```python
from build123d import *

# Parameters (mm, degrees)
F1_DEPTH = 25.4
F2_W     = 20.0148001313
F2_H     = 42.0691836625
F3_DEPTH = 25.4


with BuildPart() as f1:
    # F0 (on Top) → F1 (new body)
    with BuildSketch(Plane.XY):
        with BuildLine():
            Line((2.726720646, 50.0040240586), (2.726720646, -58.5763193667))
            Line((2.726720646, -58.5763193667), (62.9542395473, -58.5763193667))
            Line((62.9542395473, -58.5763193667), (62.9542395473, 27.6013473304))
            ThreePointArc((62.9542395473, 27.6013473304), (47.113154916, 34.1629394274), (40.5515628191, 50.0040240586))
            Line((40.5515628191, 50.0040240586), (2.726720646, 50.0040240586))
        make_face()
        with BuildLine():
            ThreePointArc((40.5515628191, 50.0040240586), (47.113154916, 34.1629394274), (62.9542395473, 27.6013473304))
            Line((62.9542395473, 27.6013473304), (62.9542395473, 50.0040240586))
            Line((62.9542395473, 50.0040240586), (40.5515628191, 50.0040240586))
        make_face()
        with BuildLine():
            Line((62.9542395473, 50.0040240586), (62.9542395473, 27.6013473304))
            ThreePointArc((62.9542395473, 27.6013473304), (78.7953241785, 34.1629394274), (85.3569162754, 50.0040240586))
            ThreePointArc((85.3569162754, 50.0040240586), (62.9542395473, 72.4067007867), (40.5515628191, 50.0040240586))
            Line((40.5515628191, 50.0040240586), (62.9542395473, 50.0040240586))
        make_face()
    extrude(amount=F1_DEPTH)

    # F2 (on face) → F3 (join)
    with BuildSketch(Plane.XY.offset(25.4)):
        with Locations((44.1186800599, 3.4223971888)):
            Rectangle(F2_W, F2_H)
    extrude(amount=F3_DEPTH)


solid = f1.part
```
Geometry: final body of the model. Coordinates: model frame, mm. A direction names the side the tool comes from. Coordinates: 2 decimals unless noted, no trailing zeros. Order: outer loops, then holes, each group sorted by start corner. A loop starts at its lowest first (then second) coordinate and runs counter-clockwise, first axis right, second up. Notation, with made-up numbers: (-12, -27) - (44, -27) arc R26 ccw to (44, -8) - close; hole circle Ø5 at (1.5, 61.25). An arc over 180 degrees is marked (long way). Write each question's results on one line, items separated by ' | '.
1) Pin query (flat end, axial travel): pin 1 (10 mm diameter, centred on x = 72.5, z = 7, fed in from -Y); pin 2 (12 mm diameter, centred on x = 32, y = -45, fed in from +Z); pin 3 (8 mm diameter, centred on y = -23, z = 38.5, fed in from -X); pin 4 (1 mm diameter, centred on x = 71.5, z = 12, fed in from +Y). Return the tip coordinate at first contact, or that it passes through.
Results list:
pin 1: y = 28.07 | pin 2: z = 25.4 | pin 3: through | pin 4: y = 70.91
2) Set-up query: faces 1 (the flat face through (54.126, 3, 38)), 2 (the flat face through (44, 24.457, 38)), 3 (the flat face through (22, 50.004, 13)), 4 (the flat face through (62.954, -16, 13)). Return all of +Z, -Z, +X, -X, +Y, -Y with unobstructed straight access to the full face (end or side cutting, diameter ignored); none if empty.
Results list:
face 1: +Z, +X, +Y, -Y | face 2: +Z, +X, -X, +Y | face 3: +Z, -Z, -X, +Y | face 4: +Z, -Z, +X, -Y
3) Line query: line 1 (Z direction, x = 70, y = 41.5); line 2 (X direction, y = 6, z = 12.5); line 3 (Y direction, x = 62, z = 3). Output: solid intervals per line, ascending. Write a range as from..to.
Results list:
line 1: 0..25.4 | line 2: 2.73..62.95 | line 3: -58.58..72.39
4) Section D-D, the plane z = 33. Return loops of the section in (x, y).
Results list:
outline: (34.11, -17.61) - (54.13, -17.61) - (54.13, 24.46) - (34.11, 24.46) - close
5) Section B-B, the plane x = 49.5. Return loops of the section in (y, z).
Results list:
outline: (-58.58, 0) - (67.92, 0) - (67.92, 25.4) - (24.46, 25.4) - (24.46, 50.8) - (-17.61, 50.8) - (-17.61, 25.4) - (-58.58, 25.4) - close
6) Section A-A, the plane y = 12. Return loops of the section in (x, z), plus the area to 3 significant figures.
Results list:
outline: (2.73, 0) - (62.95, 0) - (62.95, 25.4) - (54.13, 25.4) - (54.13, 50.8) - (34.11, 50.8) - (34.11, 25.4) - (2.73, 25.4) - close | area: 2,040 mm^2
7) Section C-C, the plane z = 6. Return loops of the section in (x, y), plus the area to 3 significant figures.
Results list:
outline: (2.73, -58.58) - (62.95, -58.58) - (62.95, 27.6) arc R22.4 ccw (long way) to (40.55, 50) - (2.73, 50) - close | area: 7,720 mm^2
